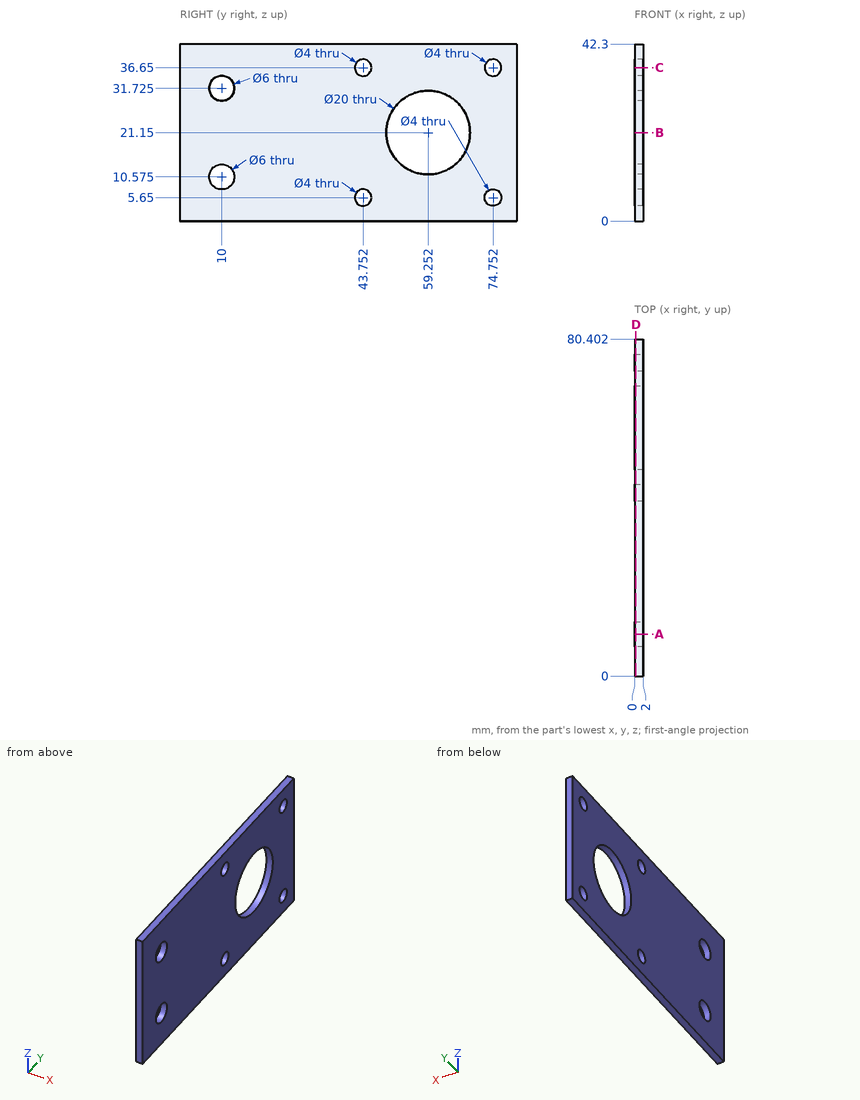
Verification items for this drawing (mm, ordinates from the low corner). Give positions to 0.01 mm unless a question says otherwise; leave off trailing zeros. Write each loop counter-clockwise with the first axis right and the second up, starting at its lowest first coordinate (ties: lowest second). Pieces come first, ordered by that corner, then holes. Notation, with made-up numbers: (59.25, 59) -> (97.25, 59) arc R30 cw to (97.25, 94) -> close; hole circle Ø8 at (-39.75, -8.75). An arc over 180 degrees is marked (long way). Use one line per item in the form item = value.
Item 1: Sectioned sample at A-A on y = 10. Enter the section's corners in (x, z) (3 decimals), plus the area to 3 significant figures.
Results list:
outline = (0, 0) -> (2, 0) -> (2, 7.575) -> (0, 7.575) -> close; (0, 13.575) -> (2, 13.575) -> (2, 28.725) -> (0, 28.725) -> close; (0, 34.725) -> (2, 34.725) -> (2, 42.3) -> (0, 42.3) -> close
area = 60.6 mm2
Item 2: Scan lines: line 1 (Z direction, x = 1.1, y = 10) (3 decimals); line 2 (Y direction, x = 0.9, z = 35.5); line 3 (Y direction, x = 0.5, z = 6). Record each from-to range of solid material in increasing order.
Results list:
line_1 = 0 to 7.575, 13.575 to 28.725, 34.725 to 42.3
line_2 = 0 to 42.12, 45.39 to 73.12, 76.39 to 80.4
line_3 = 0 to 41.78, 45.72 to 72.78, 76.72 to 80.4
Item 3: Sectioned sample at B-B on z = 21.15. Enter the section's corners in (x, y), plus the area to 3 significant figures.
Results list:
outline = (0, 0) -> (2, 0) -> (2, 49.25) -> (0, 49.25) -> close; (0, 69.25) -> (2, 69.25) -> (2, 80.4) -> (0, 80.4) -> close
area = 121 mm2
Item 4: Sectioned sample at D-D on x = 0.3. Enter the section's corners in (y, z) (3 decimals).
Results list:
outline = (0, 0) -> (80.402, 0) -> (80.402, 42.3) -> (0, 42.3) -> close; hole circle Ø6 at (10, 10.575); hole circle Ø6 at (10, 31.725); hole circle Ø4 at (43.752, 5.65); hole circle Ø4 at (43.752, 36.65); hole circle Ø20 at (59.252, 21.15); hole circle Ø4 at (74.752, 5.65); hole circle Ø4 at (74.752, 36.65)
Item 5: Sectioned sample at C-C on z = 36.65. Enter the section's corners in (x, y).
Results list:
outline = (0, 0) -> (2, 0) -> (2, 41.75) -> (0, 41.75) -> close; (0, 45.75) -> (2, 45.75) -> (2, 72.75) -> (0, 72.75) -> close; (0, 76.75) -> (2, 76.75) -> (2, 80.4) -> (0, 80.4) -> close
Item 6: Depth check by flat-ended pin: pin 1 Ø5.5 at (y, z) = (10, 31.725) entering from -X; pin 2 Ø8 at (y, z) = (46, 31.5) entering from -X. Enter the tip coordinate at first touch or a pass-through.
Results list:
pin_1 = through
pin_2 = 0
